Can you work these out from the drawing? Everything is in mm from the part's minimum corner. A direction names the side the tool comes from. Coordinates: 2 decimals unless noted, no trailing zeros. Order: outer loops, then holes, each group sorted by start corner. A loop starts at its lowest first (then second) coordinate and runs counter-clockwise, first axis right, second up. Notation, with made-up numbers: (10.25, 46) -> (61.25, 46) arc R22 ccw to (61.25, 83) -> close; hole circle Ø2 at (54.5, -37.75). An arc over 180 degrees is marked (long way). Return JSON: item names as keys, results as strings. Group by question number.
1) Thinking about a two-plate mould opening in Y: for the marked faces 3, 4, 5 and 6, which applies, +Y half, -Y half, draft (parallel to the pull), parting line (faces both ways), or undercut?
2) If we section it at C-C, the plane x = 18: Please give me the cut outline in (y, z).
3) If I drill on probe 1 along X at (y, z) = (6, 1.55); probe 2 along X at (y, z) = (49, 2); probe 3 along Y at (x, z) = (18, 2.4), over which ranges is the centre line in solid material (lowest first)? Write a range as from..to.
4) If we section it at A-A, the plane z = 27: Please give me the cut outline in (x, y).
5) For pin 1 (13 mm diameter, centred on y = 22.5, z = 21.5, fed in from -X); pin 2 (5.5 mm diameter, centred on x = 18, y = 6, fed in from +Z); pin 3 (10 mm diameter, centred on x = 4, y = 41.5, fed in from +Z), each with a flat end and sliding along its axis, tell me the tip position at first contact or that it passes through.
6) If we section it at B-B, the plane y = 27.5: Please give me the cut outline in (x, z).
7) If we section it at D-D, the plane x = 26: Please give me the cut outline in (y, z), then the cut area to 3 significant figures.
8) For the marked faces 1 and 2, which set-ups out of +Z, -Z, +X, -X, +Y, -Y let a thin tool reach every point of the face, with its end or its side?
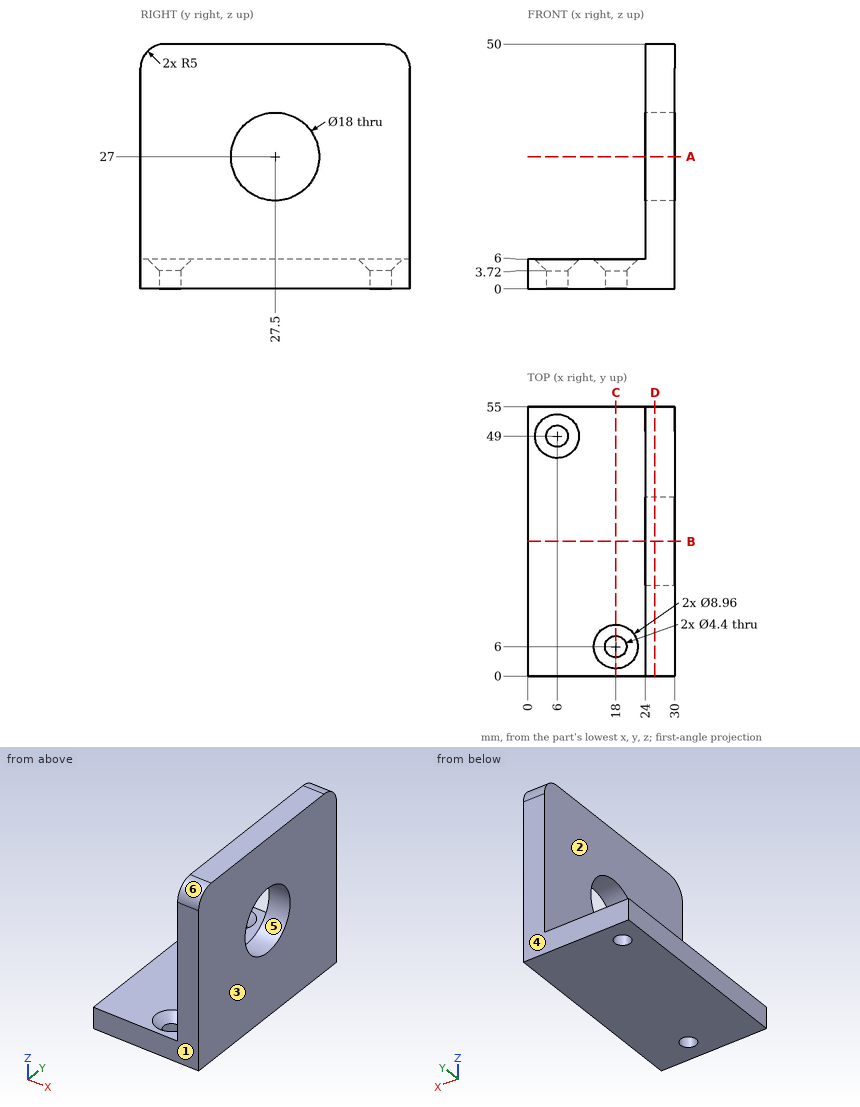
Result sheet:
{
 "1": {"face 3": "draft", "face 4": "+Y half", "face 5": "undercut", "face 6": "-Y half"},
 "2": {"outline": "(0, 0) -> (3.8, 0) -> (3.8, 3.72) -> (1.52, 6) -> (0, 6) -> close; (8.2, 0) -> (55, 0) -> (55, 6) -> (10.48, 6) -> (8.2, 3.72) -> close"},
 "3": {"probe 1": "x = 0..15.8, 20.2..30", "probe 2": "x = 0..3.8, 8.2..30", "probe 3": "y = 0..3.8, 8.2..55"},
 "4": {"outline": "(24, 0) -> (30, 0) -> (30, 18.5) -> (24, 18.5) -> close; (24, 36.5) -> (30, 36.5) -> (30, 55) -> (24, 55) -> close"},
 "5": {"pin 1": "stops at x = 24", "pin 2": "stops at z = 4.27", "pin 3": "stops at z = 6"},
 "6": {"outline": "(0, 0) -> (30, 0) -> (30, 18) -> (24, 18) -> (24, 6) -> (0, 6) -> close; (24, 36) -> (30, 36) -> (30, 50) -> (24, 50) -> close"},
 "7": {"outline": "(0, 0) -> (55, 0) -> (55, 45) arc R5 ccw to (50, 50) -> (5, 50) arc R5 ccw to (0, 45) -> close; hole circle Ø18 at (27.5, 27)", "area": "2,480 mm2"},
 "8": {"face 1": "+Z, -Z, +X, -X, -Y", "face 2": "+Z, -X, +Y, -Y"}
}
